Input: part model. Units: mm. Frame: model coordinates. Give positions to 0.01 mm unless a question says otherwise; leave off trailing zeros. Loops run counter-clockwise (first coordinate to the right, second up) from the corner with the lowest first, then second, coordinate; pieces in that order, holes last. Notation, with made-up numbers: (2.25, 40.25) -> (15.25, 40.25) arc R30 cw to (15.25, 65.25) -> close; hole circle Ø3 at (-23, 29). An arc over 180 degrees is marked (long way). Answer in a Markdown table with one row per item. Add a question column.
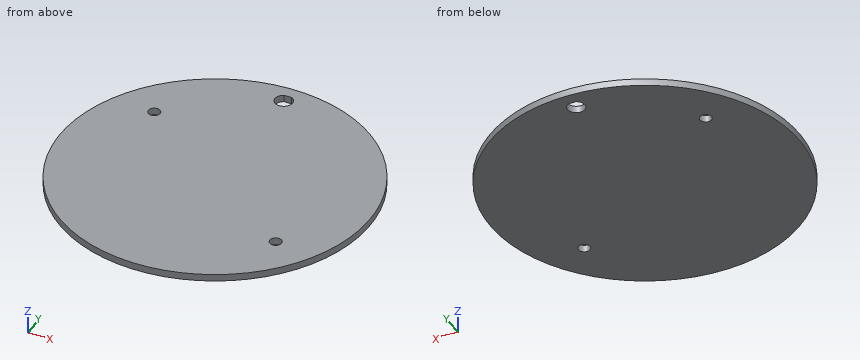
```python
from build123d import *

# Parameters (mm, degrees)
ESQUISSE1_R             = 55
BOSS_EXTRU_1_DEPTH      = 2.5
ESQUISSE2_R             = 2.1
ENL_V_MAT_EXTRU_1_DEPTH = 78.821912081
ENL_V_MAT_EXTRU_2_DEPTH = 10


with BuildPart() as part:
    # Esquisse1 → Boss.-Extru.1 (new body)
    with BuildSketch(Plane.XY):
        Circle(ESQUISSE1_R)
    extrude(amount=BOSS_EXTRU_1_DEPTH)

    # Esquisse2 → Enlèv. mat.-Extru.1 (cut, through all)
    with BuildSketch(Plane.XY.offset(2.5)):
        with Locations((33.959943273, -23.5374475)):
            Circle(ESQUISSE2_R)
        with Locations((-33.959943273, 23.5374475)):
            Circle(ESQUISSE2_R)
    extrude(amount=-ENL_V_MAT_EXTRU_1_DEPTH, mode=Mode.SUBTRACT)

    # Esquisse3 → Enlèv. mat.-Extru.2 (cut)
    with BuildSketch(Plane.XY.offset(2.5)):
        with BuildLine():
            Line((1.33041347, 50.8), (-1.33041347, 50.8))
            ThreePointArc((-1.33041347, 50.8), (0, 44.9), (1.33041347, 50.8))
        make_face()
    extrude(amount=-ENL_V_MAT_EXTRU_2_DEPTH, mode=Mode.SUBTRACT)


solid = part.part
```
1) Section D-D on x = -12.5. Output: boundary loops of the cut face in (y, z), and give its area (3 significant figures).
2) Pin query (flat end, axial travel): pin 1 (4 mm diameter, centred on x = 33.96, y = -23.54, fed in from +Z); pin 2 (1.2 mm diameter, centred on x = -0.5, z = 1, fed in from -Y). Return the tip coordinate at first contact, or that it passes through.
3) Section C-C on z = 1.25. Output: boundary loops of the cut face in (x, y), and give its area (3 significant figures).
4) Section A-A on x = 0. Output: boundary loops of the cut face in (y, z), and give its area (3 significant figures).
5) Material intervals for line 1 along Y through (x, z) = (1, 1.8); line 2 along X through (y, z) = (48, 1.9); line 3 along X through (y, z) = (45.5, 2.3), sorted ascending.
6) Section B-B on y = 47.5. Output: boundary loops of the cut face in (x, z), and give its area (3 significant figures).
Working result:
| question | item | result |
|---|---|---|
| 1 | outline | (-53.56, 0) -> (53.56, 0) -> (53.56, 2.5) -> (-53.56, 2.5) -> close |
| 1 | area | 268 mm2 |
| 2 | pin 1 | passes through |
| 2 | pin 2 | stops at y = -55 |
| 3 | outline | circle Ø110 at (0, 0); hole circle Ø4.2 at (-33.96, 23.54); hole (-1.33, 50.8) arc R3.1 ccw (long way) to (1.33, 50.8) -> close; hole circle Ø4.2 at (33.96, -23.54) |
| 3 | area | 9,450 mm2 |
| 4 | outline | (-55, 0) -> (44.9, 0) -> (44.9, 2.5) -> (-55, 2.5) -> close; (50.8, 0) -> (55, 0) -> (55, 2.5) -> (50.8, 2.5) -> close |
| 4 | area | 260 mm2 |
| 5 | line 1 | y = -54.99 to 45.07, 50.8 to 54.99 |
| 5 | line 2 | x = -26.85 to -3.1, 3.1 to 26.85 |
| 5 | line 3 | x = -30.9 to -1.83, 1.83 to 30.9 |
| 6 | outline | (-27.73, 0) -> (-3.06, 0) -> (-3.06, 2.5) -> (-27.73, 2.5) -> close; (3.06, 0) -> (27.73, 0) -> (27.73, 2.5) -> (3.06, 2.5) -> close |
| 6 | area | 123 mm2 |
